CAD build for the part. Positions are in the model's coordinates, mm. A direction names the side the tool comes from. Give positions to 0.01 mm unless a question says otherwise; leave off trailing zeros. Loops run counter-clockwise (first coordinate to the right, second up) from the corner with the lowest first, then second, coordinate; pieces in that order, holes last.
Item 1: Drop flat-ended pins along their axis: P1, Ø3.5, axis at x = 21.5, y = 25, coming from the +Z side; P2, Ø8, axis at x = 36.5, y = -34, coming from the +Z side; P3, Ø2.5, axis at x = 41.5, z = 6, coming from the -Y side. Give the stop position or say it passes through.
Item 2: Saw through at B-B on z = 5. Give the cut face in (x, y).
Item 3: Saw through at C-C on y = -25. Give the cut face in (x, z), plus the area to 3 significant figures.
Item 4: Probe probe 1 along X at (y, z) = (-29.5, 11); probe 2 along X at (y, z) = (17.5, 15.25); probe 3 along Y at (x, z) = (20, 17.6). List the from-to ranges inside material, lowest first.
Item 5: Mould opens along Y. For faces 5 (the flat face through (-52, -10, 6)), 6 (the cylindrical face through (-24.76, 21.35, 17.51)), 7 (the cylindrical face through (68, -49, 6)) say: released by +Y, released by -Y, zero draft, split by the parting line, or undercut.
Item 6: Saw through at D-D on y = 0. Give the number of separate pieces and of enclosed holes in the cut face, plus the area to 3 significant figures.
Item 7: Saw through at A-A on x = 0. Give the cut face in (y, z).
Item 8: Which spindle directions (+Z, -Z, +X, -X, +Y, -Y) get a long thin tool onto all of the face, cutting with end or side? Do faces 1 (the flat face through (-20, 25, 17)), 2 (the cylindrical face through (30.39, -46.58, 6.41)), 3 (the cylindrical face through (-43, 32, 17)), 4 (the flat face through (-1, 12, 0)). Say none if no direction does.
from build123d import *

# Parameters (mm, degrees)
F0_R     = 5
F1_DEPTH = 18
F2_R     = 6
F3_DEPTH = 1
F4_R     = 5


with BuildPart() as f1:
    # F0 (on Top) → F1 (new body)
    with BuildSketch(Plane.XY):
        with BuildLine():
            Line((0, -50), (22, -50))
            ThreePointArc((22, -50), (30.4852813742, -46.4852813742), (34, -38))
            Line((34, -38), (34, 25))
            ThreePointArc((34, 25), (35.4644660941, 28.5355339059), (39, 30))
            Line((39, 30), (47, 30))
            ThreePointArc((47, 30), (50.5355339059, 28.5355339059), (52, 25))
            Line((52, 25), (52, -45))
            ThreePointArc((52, -45), (53.4644660941, -48.5355339059), (57, -50))
            Line((57, -50), (65, -50))
            ThreePointArc((65, -50), (68.5355339059, -48.5355339059), (70, -45))
            Line((70, -45), (70, 38))
            ThreePointArc((70, 38), (66.4852813742, 46.4852813742), (58, 50))
            Line((58, 50), (0, 50))
            Line((0, 50), (-58, 50))
            ThreePointArc((-58, 50), (-66.4852813742, 46.4852813742), (-70, 38))
            Line((-70, 38), (-70, -45))
            ThreePointArc((-70, -45), (-68.5355339059, -48.5355339059), (-65, -50))
            Line((-65, -50), (-57, -50))
            ThreePointArc((-57, -50), (-53.4644660941, -48.5355339059), (-52, -45))
            Line((-52, -45), (-52, 25))
            ThreePointArc((-52, 25), (-50.5355339059, 28.5355339059), (-47, 30))
            Line((-47, 30), (-39, 30))
            ThreePointArc((-39, 30), (-35.4644660941, 28.5355339059), (-34, 25))
            Line((-34, 25), (-34, -38))
            ThreePointArc((-34, -38), (-30.4852813742, -46.4852813742), (-22, -50))
            Line((-22, -50), (0, -50))
        make_face()
        Circle(F0_R, mode=Mode.SUBTRACT)
    extrude(amount=F1_DEPTH)

    # F2 (on face) → F3 (cut)
    with BuildSketch(Plane.XY.offset(18)):
        with Locations((20, 0)):
            Circle(F2_R)
        with Locations((20, 25)):
            Circle(F2_R)
        with Locations((20, -25)):
            Circle(F2_R)
        with Locations((-20, 25)):
            Circle(F2_R)
        with Locations((-20, 0)):
            Circle(F2_R)
        with Locations((-20, -25)):
            Circle(F2_R)
    extrude(amount=-F3_DEPTH, mode=Mode.SUBTRACT)

    # F4
    f4_edges = [f1.edges().sort_by_distance(p)[0] for p in [
        (70, -3.5, 18),
    ]]
    fillet(f4_edges, radius=F4_R)


solid = f1.part
Results below:
1. P1: stops at z = 17
1. P2: stops at z = 16.57
1. P3: stops at y = 30
2. outline: (-70, -45) arc R5 ccw to (-65, -50) - (-57, -50) arc R5 ccw to (-52, -45) - (-52, 25) arc R5 cw to (-47, 30) - (-39, 30) arc R5 cw to (-34, 25) - (-34, -38) arc R12 ccw to (-22, -50) - (22, -50) arc R12 ccw to (34, -38) - (34, 25) arc R5 cw to (39, 30) - (47, 30) arc R5 cw to (52, 25) - (52, -45) arc R5 ccw to (57, -50) - (65, -50) arc R5 ccw to (70, -45) - (70, 38) arc R12 ccw to (58, 50) - (-58, 50) arc R12 ccw to (-70, 38) - close; hole circle Ø10 at (0, 0)
3. outline: (-70, 0) - (-52, 0) - (-52, 13) arc R5 ccw to (-57, 18) - (-65, 18) arc R5 ccw to (-70, 13) - close; (-34, 0) - (34, 0) - (34, 13) arc R5 ccw to (29, 18) - (26, 18) - (26, 17) - (14, 17) - (14, 18) - (-14, 18) - (-14, 17) - (-26, 17) - (-26, 18) - (-29, 18) arc R5 ccw to (-34, 13) - close; (52, 0) - (70, 0) - (70, 13) arc R5 ccw to (65, 18) - (57, 18) arc R5 ccw to (52, 13) - close
3. area: 1,820 mm2
4. probe 1: x = -70 to -52, -34 to 34, 52 to 70
4. probe 2: x = -69.47 to -52.53, -33.47 to 33.47, 52.53 to 69.47
4. probe 3: y = -46.96 to -31, -19 to -6, 6 to 19, 31 to 46.96
5. face 5: zero draft
5. face 6: undercut
5. face 7: released by -Y
6. separate pieces: 4
6. enclosed holes: 0
6. area: 1,640 mm2
7. outline: (-50, 0) - (-5, 0) - (-5, 18) - (-45, 18) arc R5 ccw to (-50, 13) - close; (5, 0) - (50, 0) - (50, 13) arc R5 ccw to (45, 18) - (5, 18) - close
8. face 1: +Z
8. face 2: +Z, -Z, -Y
8. face 3: +Z, -Y
8. face 4: -Z, +X, -X, +Y, -Y
